from build123d import *

# Parameters (mm, degrees)
SKETCH1_R           = 38.1
BOSS_EXTRUDE1_DEPTH = 12.7
SKETCH2_R           = 15.875
CUT_EXTRUDE1_DEPTH  = 9.525
SKETCH3_R           = 2.0193
CUT_EXTRUDE2_DEPTH  = 12.7
CIRPATTERN1_COUNT   = 3
CUT_EXTRUDE3_START  = -38.1
SKETCH4_R           = 2.5527
CUT_EXTRUDE3_DEPTH  = 22.431581
CIRPATTERN2_COUNT   = 3
FILLET1_R           = 0.508
SKETCH5_R           = 4.7625
SKETCH5_R_2         = 3.8735
CUT_EXTRUDE4_DEPTH  = 0.4445
CIRPATTERN3_COUNT   = 3


with BuildPart() as part:
    # Sketch1 → Boss-Extrude1 (new body)
    with BuildSketch(Plane(origin=(0, 0, 0), x_dir=(1, 0, 0), z_dir=(0, 1, 0))):
        Circle(SKETCH1_R)
    extrude(amount=BOSS_EXTRUDE1_DEPTH)

    # Sketch2 → Cut-Extrude1 (cut)
    with BuildSketch(Plane.XZ):
        Circle(SKETCH2_R)
    extrude(amount=-CUT_EXTRUDE1_DEPTH, mode=Mode.SUBTRACT)

    # Sketch3 → Cut-Extrude2 (cut)
    with BuildSketch(Plane.XZ):
        with Locations((0, 25.4)):
            Circle(SKETCH3_R)
    cut_extrude2 = extrude(amount=-CUT_EXTRUDE2_DEPTH, mode=Mode.SUBTRACT)

    # CirPattern1: Cut-Extrude2 ×3 about axis
    cirpattern1_axis = Axis((0, 0, 0), (0, 1, 0))
    for i in range(1, CIRPATTERN1_COUNT):
        add(cut_extrude2.rotate(cirpattern1_axis, i * 360 / CIRPATTERN1_COUNT), mode=Mode.SUBTRACT)

    # Sketch4 → Cut-Extrude3 (cut)
    with BuildSketch(Plane.XY.offset(CUT_EXTRUDE3_START)):
        with Locations((0, 4.7625)):
            Circle(SKETCH4_R)
    cut_extrude3 = extrude(amount=CUT_EXTRUDE3_DEPTH, mode=Mode.SUBTRACT)

    # CirPattern2: Cut-Extrude3 ×3 about axis
    cirpattern2_axis = Axis((0, 0, 0), (0, 1, 0))
    for i in range(1, CIRPATTERN2_COUNT):
        add(cut_extrude3.rotate(cirpattern2_axis, i * 360 / CIRPATTERN2_COUNT), mode=Mode.SUBTRACT)

    # Fillet1
    fillet1_edges = [part.edges().sort_by_distance(p)[0] for p in [
        (-38.1, 0, 0),
        (-38.1, 12.7, 0),
        (-15.875, 0, 0),
    ]]
    fillet(fillet1_edges, radius=FILLET1_R)

    # Sketch5 → Cut-Extrude4 (cut)
    with BuildSketch(Plane(origin=(0, 12.7, 0), x_dir=(1, 0, 0), z_dir=(0, 1, 0))):
        with Locations((0, -25.4)):
            Circle(SKETCH5_R)
        with Locations((0, -25.4)):
            Circle(SKETCH5_R_2, mode=Mode.SUBTRACT)
    cut_extrude4 = extrude(amount=-CUT_EXTRUDE4_DEPTH, mode=Mode.SUBTRACT)

    # CirPattern3: Cut-Extrude4 ×3 about axis
    cirpattern3_axis = Axis((0, 0, 0), (0, 1, 0))
    for i in range(1, CIRPATTERN3_COUNT):
        add(cut_extrude4.rotate(cirpattern3_axis, i * 360 / CIRPATTERN3_COUNT), mode=Mode.SUBTRACT)


solid = part.part
Model file for the job. Use its own axes, mm. A direction names the side the tool comes from. Coordinates: 2 decimals unless noted, no trailing zeros. Loops run counter-clockwise (first coordinate to the right, second up) from the corner with the lowest first, then second, coordinate; pieces in that order, holes last. Notation, with made-up numbers: (-26, 51) -> (-10, 51) arc R24 cw to (-10, 64) -> close; hole circle Ø7 at (69, -38). An arc over 180 degrees is marked (long way). Use one line per item in the form item = value. Start each with the question number.
(1) Flat gauge pins, fed straight in: pin 1 (5.5 mm diameter, centred on x = -22, z = -12.7, fed in from -Y); pin 2 (1 mm diameter, centred on x = 16, y = 7, fed in from +Z); pin 3 (3 mm diameter, centred on x = 0, z = 25.4, fed in from -Y); pin 4 (16 mm diameter, centred on x = -1.5, z = 4, fed in from -Y) (3 decimals). Where does each tip first touch, or does it go through?
(2) Cut at B-B on x = 0. Give the number of separate pieces and of enclosed holes in the cut face, and give its area (3 significant figures).
(3) Cut at A-A on z = 0. Give the cut face in (x, y) (3 decimals).
(4) Tool access for faces 4 (the flat face through (-20, 12.7, -11)), 5 (the cylindrical face through (-0.62, 12.48, 20.68)), 6 (the flat face through (0, 9.525, 0)): list every direction of +Z, -Z, +X, -X, +Y, -Y with a clear straight run to the whole face (end or side of a thin tool).
(5) Pull direction Y, two halves, no side cores. Call faces 1 (the cylindrical face through (-0.263, 6.261, 27.402)), 2 (the flat face through (-1, 12.7, -1)), 3 (the cylindrical face through (24.359, 6.488, 11.891)): pulls with the +Y half, pulls with the -Y half, needs draft (parallel to the pull), parting line crosses it, or undercut.
(6) Cut at D-D on y = 10.5. Give the cut face in (x, z), and give its area (3 significant figures).
(7) Probe probe 1 along Z at (x, y) = (-21, 3.5); probe 2 along Z at (x, y) = (0, 3) (3 decimals); probe 3 along Y at (x, z) = (6.5, -7) (3 decimals). List the from-to ranges inside material, lowest first. Write a range as from..to.
Values:
q1.pin_1 = 0
q1.pin_2 = 34.8
q1.pin_3 = through
q1.pin_4 = 9.525
q2.separate_pieces = 3
q2.enclosed_holes = 0
q2.area = 499 mm2
q3.outline = (-38.1, 0.508) arc R0.508 ccw to (-37.592, 0) -> (-16.383, 0) arc R0.508 ccw to (-15.875, 0.508) -> (-15.875, 9.525) -> (15.875, 9.525) -> (15.875, 0.508) arc R0.508 ccw to (16.383, 0) -> (37.592, 0) arc R0.508 ccw to (38.1, 0.508) -> (38.1, 12.192) arc R0.508 ccw to (37.592, 12.7) -> (-37.592, 12.7) arc R0.508 ccw to (-38.1, 12.192) -> close
q4.face_4 = +Z, -Z, +X, -X, +Y
q4.face_5 = +Y
q4.face_6 = -Y
q5.face_1 = needs draft
q5.face_2 = pulls with the +Y half
q5.face_3 = undercut
q6.outline = circle Ø76.2 at (0, 0); hole circle Ø4.04 at (-22, -12.7); hole circle Ø4.04 at (0, 25.4); hole circle Ø4.04 at (22, -12.7)
q6.area = 4,520 mm2
q7.probe_1 = -31.79..-14.46, -10.94..9.56, 14.69..31.79
q7.probe_2 = 15.875..23.381, 27.419..38.1
q7.probe_3 = 9.525..12.7
